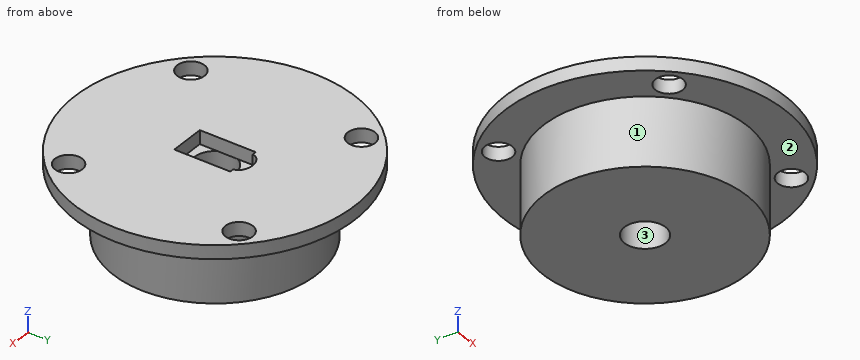
```python
from build123d import *

# Parameters (mm, degrees)
F0_R      = 20.5
F1_DEPTH  = 2
F2_R      = 14.875
F3_DEPTH  = 10
F4_R      = 2
F5_DEPTH  = 2
F6_R      = 3
F7_DEPTH  = 10
F8_W      = 5.2
F8_H      = 8.2
F9_DEPTH  = 2
F11_DEPTH = 2


with BuildPart() as f1:
    # F0 (on Top) → F1 (new body)
    with BuildSketch(Plane.XY):
        Circle(F0_R)
    extrude(amount=F1_DEPTH)

    # F2 (on Top) → F3 (join)
    with BuildSketch(Plane.XY):
        Circle(F2_R)
    extrude(amount=-F3_DEPTH)

    # F4 (on Top) → F5 (cut)
    with BuildSketch(Plane.XY):
        with Locations((-12.5, 12.5)):
            Circle(F4_R)
        with Locations((12.5, 12.5)):
            Circle(F4_R)
        with Locations((12.5, -12.5)):
            Circle(F4_R)
        with Locations((-12.5, -12.5)):
            Circle(F4_R)
    extrude(amount=F5_DEPTH, mode=Mode.SUBTRACT)

    # F6 (on Top) → F7 (cut)
    with BuildSketch(Plane.XY):
        Circle(F6_R)
    extrude(amount=-F7_DEPTH, mode=Mode.SUBTRACT)

    # F8 (on Top) → F9 (cut)
    with BuildSketch(Plane.XY):
        Rectangle(F8_W, F8_H)
    extrude(amount=F9_DEPTH, mode=Mode.SUBTRACT)

    # F10 (on Top) → F11 (cut)
    with BuildSketch(Plane.XY):
        with BuildLine():
            add(Edge.make_bspline(
                [(2, 4), (2, 6.598076), (-1, 5.299038), (-4, 4), (-1, 2.700962), (2, 1.401924), (2, 4)],
                knots=[0, 0, 0, 2.094395, 2.094395, 4.18879, 4.18879, 6.283185, 6.283185, 6.283185], degree=2, weights=[1, 0.5, 1, 0.5, 1, 0.5, 1]))
        make_face()
    extrude(amount=F11_DEPTH, mode=Mode.SUBTRACT)


solid = f1.part
```
Check sheet for the modelled part. Datum: model origin and axes. Units: mm. Face numbers are marked on the shaded views. Give positions to 0.01 mm unless a question says otherwise; leave off trailing zeros. Order: outer loops, then holes, each group sorted by start corner. A loop starts at its lowest first (then second) coordinate and runs counter-clockwise, first axis right, second up. Notation, with made-up numbers: (86, 55) -> (121, 55) arc R18 ccw to (121, 75) -> close; hole circle Ø9 at (62, 10.25). An arc over 180 degrees is marked (long way). Return JSON: item names as keys, results as strings.
1. Cross-section at D-D, the plane z = -7. Record the cut outline in (x, y) (3 decimals), plus the area to 3 significant figures.
From the geometry:
{"outline": "circle Ø29.75 at (0, 0); hole circle Ø6 at (0, 0)", "area": "667 mm^2"}
2. Mould release check, pull along Y, two halves, no side actions. Record for the marked faces 1, 2 and 3: +Y half, -Y half, draft (parallel to the pull), parting line (faces both ways), or undercut.
From the geometry:
{"face 1": "parting line", "face 2": "draft", "face 3": "undercut"}
3. Cross-section at C-C, the plane y = 7. Record the cut outline in (x, z) (3 decimals), plus the area to 3 significant figures.
From the geometry:
{"outline": "(-19.268, 0) -> (-13.125, 0) -> (-13.125, -10) -> (13.125, -10) -> (13.125, 0) -> (19.268, 0) -> (19.268, 2) -> (-19.268, 2) -> close", "area": "340 mm^2"}
4. Cross-section at A-A, the plane y = -12.5. Record the cut outline in (x, z), plus the area to 3 significant figures.
From the geometry:
{"outline": "(-16.25, 0) -> (-14.5, 0) -> (-14.5, 2) -> (-16.25, 2) -> close; (-10.5, 0) -> (-8.06, 0) -> (-8.06, -10) -> (8.06, -10) -> (8.06, 0) -> (10.5, 0) -> (10.5, 2) -> (-10.5, 2) -> close; (14.5, 0) -> (16.25, 0) -> (16.25, 2) -> (14.5, 2) -> close", "area": "210 mm^2"}
5. Material ranges on probe 1 along Y at (x, z) = (0, -2) (3 decimals); probe 2 along Y at (x, z) = (12.5, 1.05); probe 3 along Z at (x, y) = (-10, 12), recorded low to high. Write a range as [from, to].
From the geometry:
{"probe 1": "[-14.875, -3], [3, 14.875]", "probe 2": "[-16.25, -14.5], [-10.5, 10.5], [14.5, 16.25]", "probe 3": "[0, 2]"}
6. Go/stop test with flat-tipped pins: P1, Ø1.2, axis at x = -0.5, y = 3.5, coming from the +Z side; P2, Ø2, axis at x = 14, z = -4.5, coming from the +Y side; P3, Ø1.6, axis at x = 0.5, z = 1, coming from the +Y side; P4, Ø3.5, axis at x = 12.5, y = -12.5, coming from the -Z side. Record where each tip stops, or that it passes through.
From the geometry:
{"P1": "z = 0", "P2": "y = 7.23", "P3": "y = 20.5", "P4": "through"}
